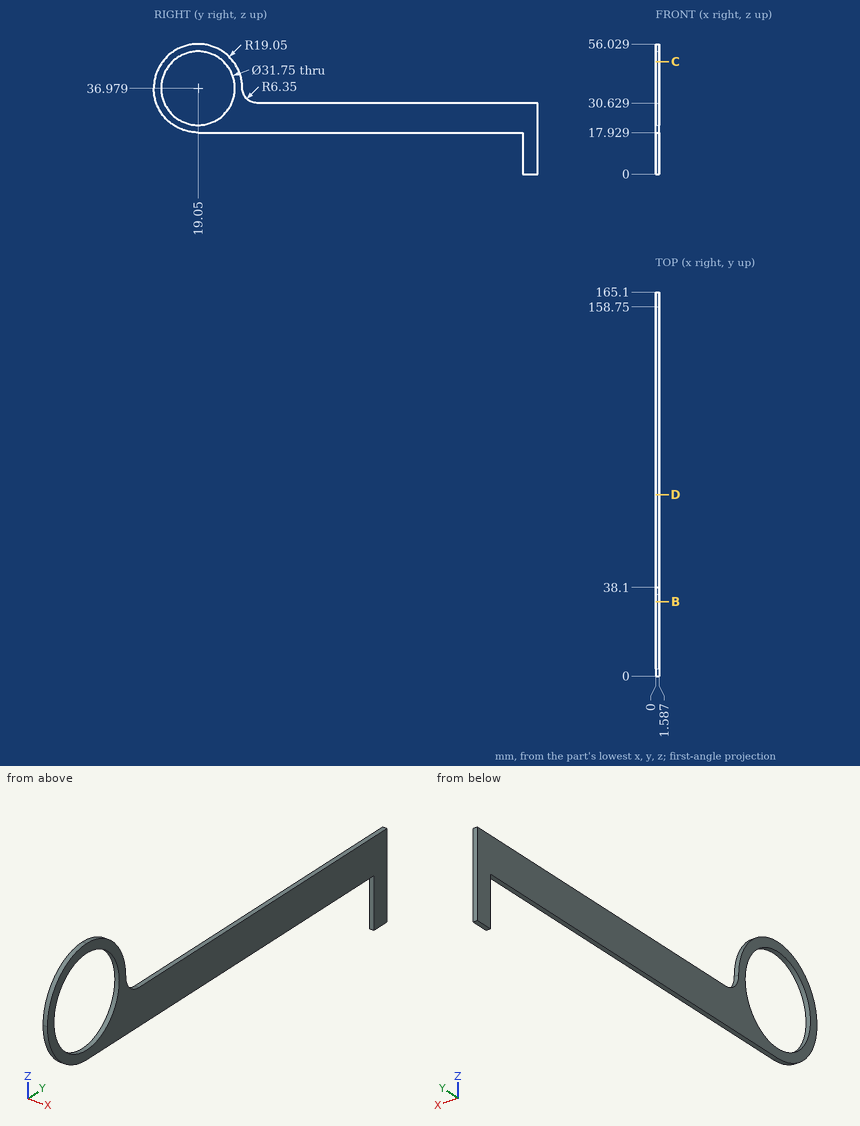
Input: dimensioned drawing with shaded views. Units: mm. Origin: part minimum x, y, z. Coordinates: 2 decimals unless noted, no trailing zeros. Write each loop counter-clockwise with the first axis right and the second up, starting at its lowest first coordinate (ties: lowest second). Pieces come first, ordered by that corner, then holes. Notation, with made-up numbers: M -6,57.25 L 6,57.25 A15 ccw 6,62.25 Z; hole C -25.5,1.25 d2. An arc over 180 degrees is marked long. Use one line per item in the form item = value.
Q1. First-contact query: pin 1 (0.8 mm diameter, centred on x = 0.5, z = 5, fed in from -Y); pin 2 (0.5 mm diameter, centred on x = 1, y = 132, fed in from +Z). Flat tips, straight axial feed; report the tip coordinate or a pass-through.
Answer below:
pin_1 = 158.75
pin_2 = 30.63
Q2. Section C-C (z = 48.5). Return loops of the section in (x, y).
Answer below:
outline = M 0,3.88 L 1.59,3.88 L 1.59,8.13 L 0,8.13 Z; M 0,29.97 L 1.59,29.97 L 1.59,34.22 L 0,34.22 Z
Q3. Material intervals for probe 1 along Z at (x, y) = (1.2, 19.05) (1 decimal); probe 2 along Y at (x, z) = (0.9, 35) (1 decimal); probe 3 along Z at (x, y) = (1.2, 126.5), sorted ascending. Write a range as from..to.
Answer below:
probe_1 = 17.9..21.1, 52.9..56
probe_2 = 0.1..3.3, 34.8..38.4
probe_3 = 17.93..30.63
Q4. Section D-D (y = 78). Return loops of the section in (x, z).
Answer below:
outline = M 0,17.93 L 1.59,17.93 L 1.59,30.63 L 0,30.63 Z
Q5. Section B-B (y = 32). Return loops of the section in (x, z).
Answer below:
outline = M 0,17.93 L 1.59,17.93 L 1.59,27.8 L 0,27.8 Z; M 0,46.16 L 1.59,46.16 L 1.59,50.95 L 0,50.95 Z
